Verification items for the finished model (mm, model axes). A direction names the side the tool comes from. Round coordinates to 2 decimals unless told otherwise and drop trailing zeros. Write each loop counter-clockwise with the first axis right and the second up, starting at its lowest first coordinate (ties: lowest second). Pieces come first, ordered by that corner, then holes. Notation, with made-up numbers: M -25.75,30 L -20.75,30 A33 ccw -20.75,68 Z; hole C -25.75,-13 d11. An arc over 180 degrees is marked long. One line per question, with ' | ' between items.
from build123d import *

# Parameters (mm, degrees)
SKETCH1_W           = 17
SKETCH1_H           = 17
BOSS_EXTRUDE1_DEPTH = 4
CHAMFER1_SIZE       = 2.5
BOSS_EXTRUDE3_DEPTH = 4
SKETCH2_R           = 9
BOSS_EXTRUDE2_DEPTH = 23


with BuildPart() as part:
    # Sketch1 → Boss-Extrude1 (new body)
    with BuildSketch(Plane.XY):
        Rectangle(SKETCH1_W, SKETCH1_H)
    extrude(amount=BOSS_EXTRUDE1_DEPTH)

    # Chamfer1
    chamfer1_edges = [part.edges().sort_by_distance(p)[0] for p in [
        (8.5, -8.5, 2),
        (-8.5, -8.5, 2),
        (-8.5, 8.5, 2),
        (8.5, 8.5, 2),
    ]]
    chamfer(chamfer1_edges, length=CHAMFER1_SIZE)

    # Sketch3 → Boss-Extrude3 (add)
    with BuildSketch(Plane.XY):
        with BuildLine():
            Line((-8.5, 2), (-9, 2))
            ThreePointArc((-9, 2), (-11, 0), (-9, -2))
            Line((-9, -2), (-8.5, -2))
            Line((-8.5, -2), (-8.5, 2))
        make_face()
    boss_extrude3 = extrude(amount=BOSS_EXTRUDE3_DEPTH)

    # Mirror1: Boss-Extrude3 across plane
    add(boss_extrude3.mirror(Plane(origin=(0, 0, 0), x_dir=(0, 0, 1), z_dir=(1, 0, 0))))

    # Sketch2 → Boss-Extrude2 (add)
    with BuildSketch(Plane.XY.offset(4)):
        Circle(SKETCH2_R)
    extrude(amount=BOSS_EXTRUDE2_DEPTH)


solid = part.part
1. Section check C-C, the plane z = 18. Record the cut outline in (x, y), then the cut area to 3 significant figures.
Results:
outline: C 0,0 d18 | area: 254 mm2
2. Section check B-B, the plane x = -7.75. Record the cut outline in (y, z).
Results:
outline: M -6.75,0 L 6.75,0 L 6.75,4 L 4.58,4 L 4.58,27 L -4.58,27 L -4.58,4 L -6.75,4 Z
3. Go/stop test with flat-tipped pins: P1, Ø2, axis at y = -3, z = 7.5, coming from the +X side; P2, Ø0.6, axis at x = -8.5, z = 1.5, coming from the +Y side; P3, Ø3, axis at x = -0.5, z = 2, coming from the +Y side. Record where each tip stops, or that it passes through.
Results:
P1: stops at x = 8.77 | P2: stops at y = 6.3 | P3: stops at y = 8.5
4. Tool access check on faces 1 (the face through (0, 8.5, 2)), 2 (the face through (7, -7, 4)), 3 (the face through (8.5, 4, 2)). Record the directions out of +Z, -Z, +X, -X, +Y, -Y that give a thin tool (end or side, any length) a straight path to the whole face; none if there is none.
Results:
face 1: -Z, +X, -X, +Y | face 2: +Z, +X, -Y | face 3: -Z, +X, +Y
5. Thickness scan on line 1 (X direction, y = 2, z = 4.5); line 2 (Z direction, x = 7.25, y = -6.5). Record the ranges inside material, lowest first.
Results:
line 1: x = -8.77 to 8.77 | line 2: z = 0 to 4
6. Section check A-A, the plane y = 0. Record the cut outline in (x, z), then the cut area to 3 significant figures.
Results:
outline: M -11,0 L 11,0 L 11,4 L 9,4 L 9,27 L -9,27 L -9,4 L -11,4 Z | area: 502 mm2
